Study the drawing (mm; zero at the part's minimum x, y, z) and answer. A direction names the side the tool comes from. Coordinates: 2 decimals unless noted, no trailing zeros. Order: outer loops, then holes, each group sorted by start corner. A loop starts at its lowest first (then second) coordinate and runs counter-clockwise, first axis right, second up.
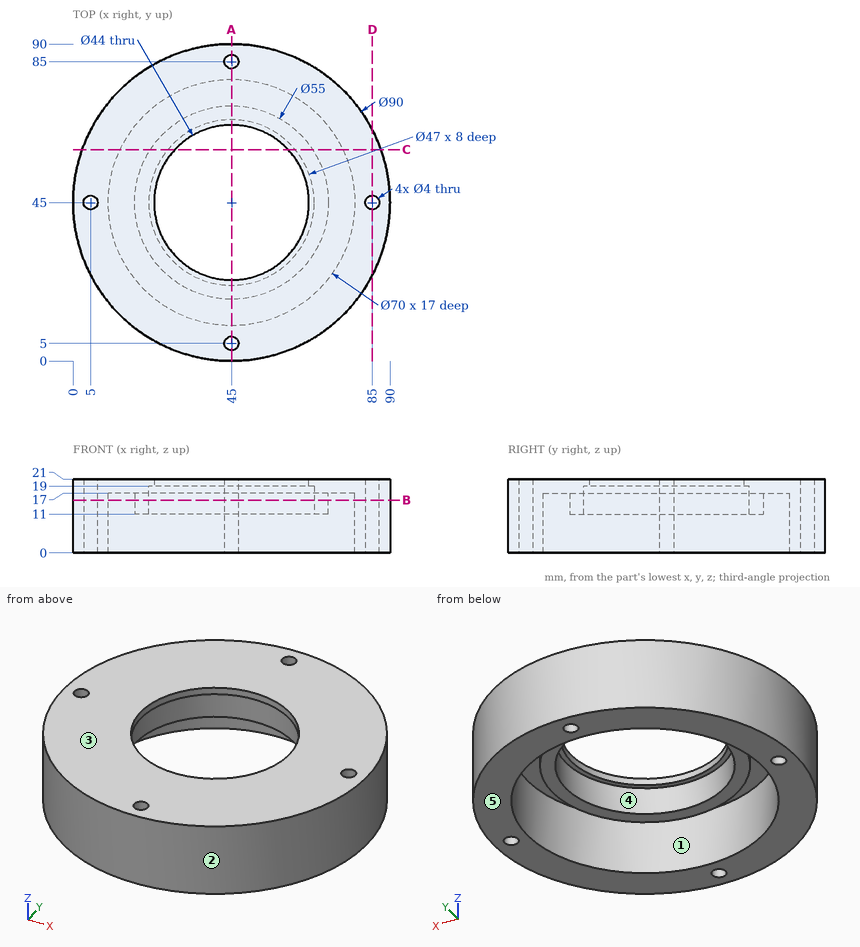
1) Straight lines are drawn through the part: line 1 (X direction, y = 45, z = 6); line 2 (Y direction, x = 45, z = 16.5); line 3 (Y direction, x = 45, z = 19.75). For each, find the intervals that lie inside material, in ascending order.
A:
line 1: x = 0 to 3, 7 to 10, 80 to 83, 87 to 90
line 2: y = 0 to 3, 7 to 10, 17.5 to 21.5, 68.5 to 72.5, 80 to 83, 87 to 90
line 3: y = 0 to 3, 7 to 23, 67 to 83, 87 to 90
2) Flat-ended cylindrical pins translate along their axes: pin 1 Ø12 at (y, z) = (73.5, 7.5) entering from -X; pin 2 Ø14 at (x, y) = (41, 56.5) entering from -Z; pin 3 Ø3 at (x, y) = (13, 52.5) entering from -Z; pin 4 Ø1 at (y, z) = (26, 8.5) entering from -X. Find the tip coordinate at first contact, or state that the pin passes through.
A:
pin 1: stops at x = 6.03
pin 2: passes through
pin 3: stops at z = 17
pin 4: stops at x = 3.98
3) A cutting plane is placed at C-C, the plane y = 60. Determine the outline of the cut face in (x, z), and give its area (3 significant figures).
A:
outline: (2.57, 0) - (13.38, 0) - (13.38, 17) - (21.95, 17) - (21.95, 11) - (26.91, 11) - (26.91, 19) - (28.91, 19) - (28.91, 21) - (2.57, 21) - close; (61.09, 19) - (63.09, 19) - (63.09, 11) - (68.05, 11) - (68.05, 17) - (76.62, 17) - (76.62, 0) - (87.43, 0) - (87.43, 21) - (61.09, 21) - close
area: 630 mm2
4) A cutting plane is placed at A-A, the plane x = 45. Determine the outline of the cut face in (y, z).
A:
outline: (0, 0) - (3, 0) - (3, 21) - (0, 21) - close; (7, 0) - (10, 0) - (10, 17) - (17.5, 17) - (17.5, 11) - (21.5, 11) - (21.5, 19) - (23, 19) - (23, 21) - (7, 21) - close; (67, 19) - (68.5, 19) - (68.5, 11) - (72.5, 11) - (72.5, 17) - (80, 17) - (80, 0) - (83, 0) - (83, 21) - (67, 21) - close; (87, 0) - (90, 0) - (90, 21) - (87, 21) - close
5) A cutting plane is placed at D-D, the plane x = 85. Determine the outline of the cut face in (y, z).
A:
outline: (24.38, 0) - (43, 0) - (43, 21) - (24.38, 21) - close; (47, 0) - (65.62, 0) - (65.62, 21) - (47, 21) - close
6) A cutting plane is placed at B-B, the plane z = 15. Determine the outline of the cut face in (x, y), and give its area (3 significant figures).
A:
outline: circle Ø90 at (45, 45); circle Ø55 at (45, 45); hole circle Ø4 at (5, 45); hole circle Ø70 at (45, 45); hole circle Ø47 at (45, 45); hole circle Ø4 at (45, 5); hole circle Ø4 at (45, 85); hole circle Ø4 at (85, 45)
area: 3,100 mm2
7) Which of the six approach directions +Z, -Z, +X, -X, +Y, -Y give full straight-line access (tool end or side, diameter ignored) to the marked faces 4 and 5?
A:
face 4: -Z
face 5: -Z, +X, -X, +Y, -Y
8) Determine the mould class of the marked faces 1, 2 and 3 for opening direction Y: pulls with the +Y half, pulls with the -Y half, needs draft (parallel to the pull), parting line crosses it, or undercut.
A:
face 1: undercut
face 2: parting line crosses it
face 3: needs draft
